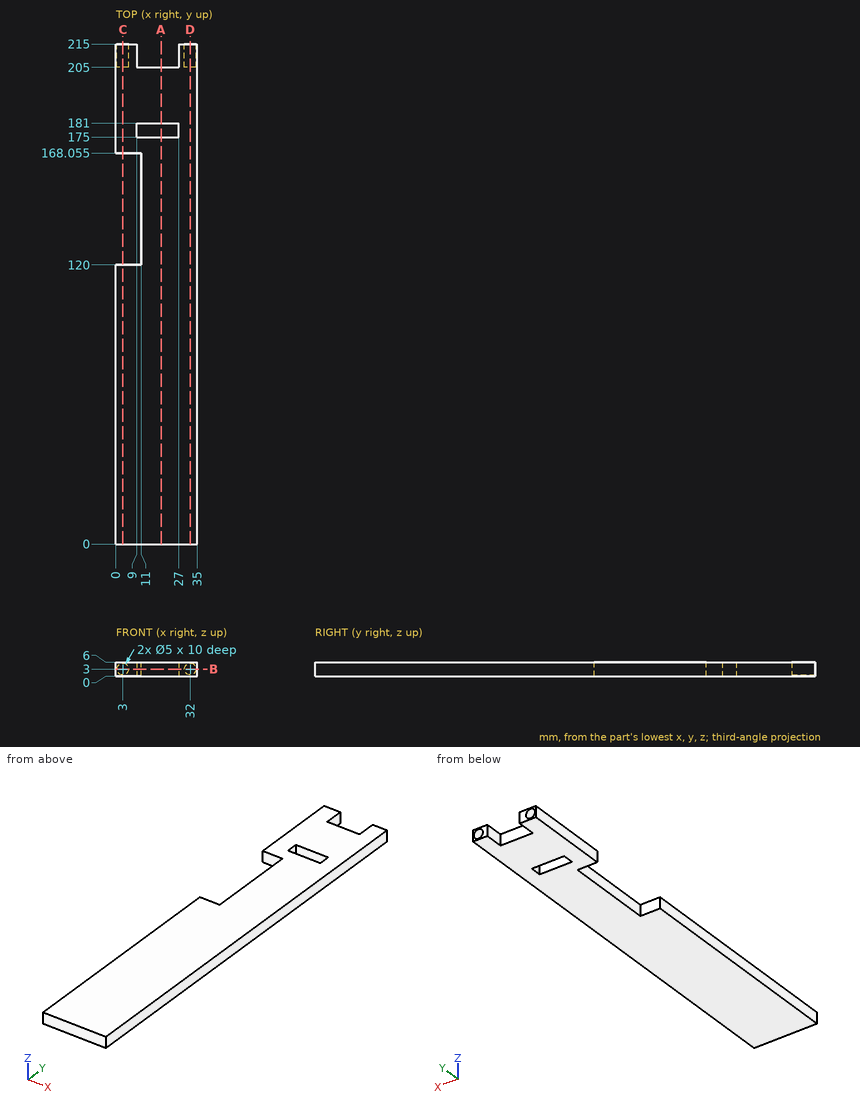
Could you check a few things on this drawing? It's one solid part, dimensions in mm from its lowest x, y, z. Coordinates: 2 decimals unless noted, no trailing zeros. Write each loop counter-clockwise with the first axis right and the second up, starting at its lowest first coordinate (ties: lowest second). Pieces come first, ordered by that corner, then holes. Notation, with made-up numbers: (68, 74) - (94, 74) arc R19 cw to (94, 102) - close; hole circle Ø9 at (33.5, -22). An arc over 180 degrees is marked (long way). Use one line per item in the form item = value.
1) Suppose I cut it at B-B, the plane z = 3. Write out the boundary of the cut face in (x, y) (1 decimal), plus the area to 3 significant figures.
Solved:
outline = (0, 0) - (35, 0) - (35, 215) - (34.5, 215) - (34.5, 205) - (29.5, 205) - (29.5, 215) - (27, 215) - (27, 205) - (9, 205) - (9, 215) - (5.5, 215) - (5.5, 205) - (0.5, 205) - (0.5, 215) - (0, 215) - (0, 168.1) - (11, 168.1) - (11, 120) - (0, 120) - close; hole (9, 175) - (27, 175) - (27, 181) - (9, 181) - close
area = 6,610 mm2
2) Suppose I cut it at A-A, the plane x = 19.5. Write out the boundary of the cut face in (y, z), plus the area to 3 significant figures.
Solved:
outline = (0, 0) - (175, 0) - (175, 6) - (0, 6) - close; (181, 0) - (205, 0) - (205, 6) - (181, 6) - close
area = 1,190 mm2
3) I need wall thicknesses on line 1 (X direction, y = 212, z = 3); line 2 (Y direction, x = 16.5, z = 5.6); line 3 (Y direction, x = 4, z = 4.2) (1 decimal). Which ranges of each line are inside material? Lowest first, please.
Solved:
line_1 = 0 to 0.5, 5.5 to 9, 27 to 29.5, 34.5 to 35
line_2 = 0 to 175, 181 to 205
line_3 = 0 to 120, 168.1 to 205
4) Suppose I cut it at C-C, the plane x = 3. Write out the boundary of the cut face in (y, z) (1 decimal).
Solved:
outline = (0, 0) - (120, 0) - (120, 6) - (0, 6) - close; (168.1, 0) - (215, 0) - (215, 0.5) - (205, 0.5) - (205, 5.5) - (215, 5.5) - (215, 6) - (168.1, 6) - close
5) Suppose I cut it at D-D, the plane x = 32. Write out the boundary of the cut face in (y, z), plus the area to 3 significant figures.
Solved:
outline = (0, 0) - (215, 0) - (215, 0.5) - (205, 0.5) - (205, 5.5) - (215, 5.5) - (215, 6) - (0, 6) - close
area = 1,240 mm2
